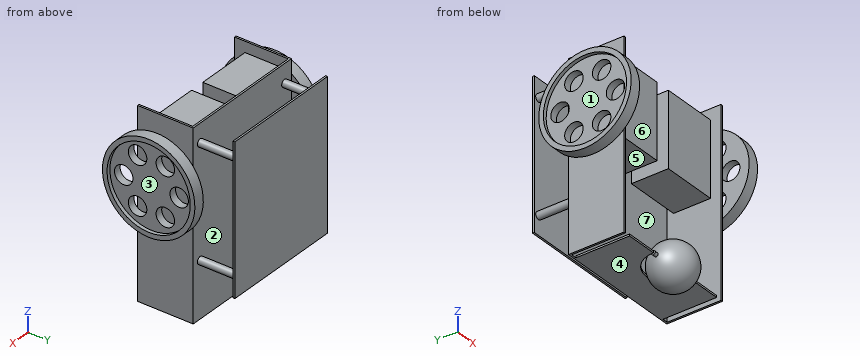
from build123d import *

# Parameters (mm, degrees)
SKETCH_1_W               = 70
SKETCH_1_H               = 100
EXTRUDE_1_DEPTH          = 30
SHELL_1_T                = -1
SKETCH_2_W               = 40
SKETCH_2_H               = 20
EXTRUDE_2_DEPTH          = 30
SKETCH_3_R               = 1.5
EXTRUDE_3_DEPTH          = 10
SKETCH_4_R               = 25
EXTRUDE_4_DEPTH          = 6
SKETCH_5_R               = 22.5
CUT_EXTRUDE_1_DEPTH      = 2
SKETCH_6_R               = 5
CUT_EXTRUDE_2_DEPTH      = 8
PATTERN_CIRCULAR_1_COUNT = 6
MIRROR_1_COPY_1_SKETCH_R = 5
MIRROR_1_COPY_1_DEPTH    = 8
MIRROR_1_COPY_2_SKETCH_R = 5
MIRROR_1_COPY_2_DEPTH    = 8
MIRROR_1_COPY_3_SKETCH_R = 5
MIRROR_1_COPY_3_DEPTH    = 8
MIRROR_1_COPY_4_SKETCH_R = 5
MIRROR_1_COPY_4_DEPTH    = 8
MIRROR_1_COPY_5_SKETCH_R = 5
MIRROR_1_COPY_5_DEPTH    = 8
SKETCH_9_R               = 14
CUT_EXTRUDE_4_DEPTH      = 8
SKETCH_8_W               = 3
SKETCH_8_H               = 29
CUT_EXTRUDE_3_DEPTH      = 8
SKETCH_10_R              = 1
EXTRUDE_5_DEPTH          = 14
SKETCH_11_R              = 2
EXTRUDE_6_DEPTH          = 20
SKETCH_12_W              = 66
SKETCH_12_H              = 80
EXTRUDE_7_DEPTH          = 1


with BuildPart() as part:
    # Sketch 1 → Extrude 1 (new body)
    with BuildSketch(Plane(origin=(0, 0, 0), x_dir=(1, 0, 0), z_dir=(0, 1, 0))):
        with Locations((0, 50)):
            Rectangle(SKETCH_1_W, SKETCH_1_H)
    extrude(amount=EXTRUDE_1_DEPTH)

    # Shell 1
    shell_1_openings = [part.faces().sort_by_distance(p)[0] for p in [
        (0, 0, -50),
        (0, 15, 0),
    ]]
    offset(amount=SHELL_1_T, openings=shell_1_openings, kind=Kind.INTERSECTION)

    # Sketch 2 → Extrude 2 (add)
    with BuildSketch(Plane.ZY.offset(-34)):
        with Locations((-25.793166275, 15.578551741)):
            Rectangle(SKETCH_2_W, SKETCH_2_H)
    extrude_2 = extrude(amount=EXTRUDE_2_DEPTH)

    # Sketch 3 → Extrude 3 (add)
    with BuildSketch(Plane(origin=(35, 0, 0), x_dir=(0, 0, -1), z_dir=(1, 0, 0))):
        with Locations((32, 13.5)):
            Circle(SKETCH_3_R)
    extrude_3 = extrude(amount=EXTRUDE_3_DEPTH)

    # Sketch 4 → Extrude 4 (add)
    with BuildSketch(Plane(origin=(45, 0, 0), x_dir=(0, 0, -1), z_dir=(1, 0, 0))):
        with Locations((32, 13.5)):
            Circle(SKETCH_4_R)
    extrude_4 = extrude(amount=-EXTRUDE_4_DEPTH)

    # Sketch 5 → Cut-Extrude 1 (cut)
    with BuildSketch(Plane(origin=(45, 0, 0), x_dir=(0, 0, -1), z_dir=(1, 0, 0))):
        with Locations((32, 13.5)):
            Circle(SKETCH_5_R)
    cut_extrude_1 = extrude(amount=-CUT_EXTRUDE_1_DEPTH, mode=Mode.SUBTRACT)

    # Sketch 6 → Cut-Extrude 2 (cut)
    with BuildSketch(Plane(origin=(43, 0, 0), x_dir=(0, 0, -1), z_dir=(1, 0, 0))):
        with Locations((32, 28.5)):
            Circle(SKETCH_6_R)
    cut_extrude_2 = extrude(amount=-CUT_EXTRUDE_2_DEPTH, mode=Mode.SUBTRACT)

    # Pattern Circular 1: Cut-Extrude 2 ×6 about axis
    pattern_circular_1_axis = Axis((0, 13.5, -32), (1, 0, 0))
    for i in range(1, PATTERN_CIRCULAR_1_COUNT):
        add(cut_extrude_2.rotate(pattern_circular_1_axis, i * 360 / PATTERN_CIRCULAR_1_COUNT), mode=Mode.SUBTRACT)

    # Mirror 1: Extrude 2, Extrude 3, Extrude 4, Cut-Extrude 1, Cut-Extrude 2 across plane
    add(extrude_2.mirror(Plane(origin=(0, 0, 0), x_dir=(0, 0, 1), z_dir=(1, 0, 0))))
    add(extrude_3.mirror(Plane(origin=(0, 0, 0), x_dir=(0, 0, 1), z_dir=(1, 0, 0))))
    add(extrude_4.mirror(Plane(origin=(0, 0, 0), x_dir=(0, 0, 1), z_dir=(1, 0, 0))))
    add(cut_extrude_1.mirror(Plane(origin=(0, 0, 0), x_dir=(0, 0, 1), z_dir=(1, 0, 0))), mode=Mode.SUBTRACT)
    add(cut_extrude_2.mirror(Plane(origin=(0, 0, 0), x_dir=(0, 0, 1), z_dir=(1, 0, 0))), mode=Mode.SUBTRACT)

    # Mirror 1 copy 1 sketch → Mirror 1 copy 1 (cut)
    with BuildSketch(Plane(origin=(-43, -20.962812921, -27.691342951), x_dir=(0, 0.866025404, -0.5), z_dir=(-1, 0, 0))):
        with Locations((32, -28.5)):
            Circle(MIRROR_1_COPY_1_SKETCH_R)
    extrude(amount=-MIRROR_1_COPY_1_DEPTH, mode=Mode.SUBTRACT)

    # Mirror 1 copy 2 sketch → Mirror 1 copy 2 (cut)
    with BuildSketch(Plane(origin=(-43, -7.462812921, -59.691342951), x_dir=(0, 0.866025404, 0.5), z_dir=(-1, 0, 0))):
        with Locations((32, -28.5)):
            Circle(MIRROR_1_COPY_2_SKETCH_R)
    extrude(amount=-MIRROR_1_COPY_2_DEPTH, mode=Mode.SUBTRACT)

    # Mirror 1 copy 3 sketch → Mirror 1 copy 3 (cut)
    with BuildSketch(Plane(origin=(-43, 27, -64), x_dir=(0, 0, 1), z_dir=(-1, 0, 0))):
        with Locations((32, -28.5)):
            Circle(MIRROR_1_COPY_3_SKETCH_R)
    extrude(amount=-MIRROR_1_COPY_3_DEPTH, mode=Mode.SUBTRACT)

    # Mirror 1 copy 4 sketch → Mirror 1 copy 4 (cut)
    with BuildSketch(Plane(origin=(-43, 47.962812921, -36.308657049), x_dir=(0, -0.866025404, 0.5), z_dir=(-1, 0, 0))):
        with Locations((32, -28.5)):
            Circle(MIRROR_1_COPY_4_SKETCH_R)
    extrude(amount=-MIRROR_1_COPY_4_DEPTH, mode=Mode.SUBTRACT)

    # Mirror 1 copy 5 sketch → Mirror 1 copy 5 (cut)
    with BuildSketch(Plane(origin=(-43, 34.462812921, -4.308657049), x_dir=(0, -0.866025404, -0.5), z_dir=(-1, 0, 0))):
        with Locations((32, -28.5)):
            Circle(MIRROR_1_COPY_5_SKETCH_R)
    extrude(amount=-MIRROR_1_COPY_5_DEPTH, mode=Mode.SUBTRACT)

    # Sketch 9 → Cut-Extrude 4 (cut)
    with BuildSketch(Plane(origin=(0, 0, -100), x_dir=(-1, 0, 0), z_dir=(0, 0, -1))):
        Circle(SKETCH_9_R)
    extrude(amount=-CUT_EXTRUDE_4_DEPTH, mode=Mode.SUBTRACT)

    # Sketch 8 → Cut-Extrude 3 (cut)
    with BuildSketch(Plane(origin=(0, 0, -100), x_dir=(-1, 0, 0), z_dir=(0, 0, -1))):
        with Locations((32.5, 14.5)):
            Rectangle(SKETCH_8_W, SKETCH_8_H)
        with Locations((-32.5, 14.5)):
            Rectangle(SKETCH_8_W, SKETCH_8_H)
    extrude(amount=-CUT_EXTRUDE_3_DEPTH, mode=Mode.SUBTRACT)



with BuildPart() as body_2:
    # Sketch 7 → Revolve 1 (revolve)
    with BuildSketch(Plane(origin=(0, 0, -100), x_dir=(-1, 0, 0), z_dir=(0, 0, -1))):
        with BuildLine():
            Line((-12, 0), (12, 0))
            ThreePointArc((12, 0), (0, 12), (-12, 0))
        make_face()
    revolve(axis=Axis((12, 0, -100), (-1, 0, 0)))


with BuildPart() as part_1:
    add(part.part)

    add(body_2.part)  # Extrude 5 merges body 2
    # Sketch 10 → Extrude 5 (add, symmetric)
    with BuildSketch(Plane(origin=(0, 0, 0), x_dir=(0, 0, -1), z_dir=(1, 0, 0))):
        with Locations((100, 0)):
            Circle(SKETCH_10_R)
    extrude(amount=EXTRUDE_5_DEPTH, both=True)

    # Sketch 11 → Extrude 6 (add)
    with BuildSketch(Plane(origin=(0, 30, 0), x_dir=(1, 0, 0), z_dir=(0, 1, 0))):
        with Locations((30, 70)):
            Circle(SKETCH_11_R)
        with Locations((-30, 70)):
            Circle(SKETCH_11_R)
        with Locations((-30, 10)):
            Circle(SKETCH_11_R)
        with Locations((30, 10)):
            Circle(SKETCH_11_R)
    extrude(amount=EXTRUDE_6_DEPTH)

    # Sketch 12 → Extrude 7 (add)
    with BuildSketch(Plane(origin=(0, 50, 0), x_dir=(1, 0, 0), z_dir=(0, 1, 0))):
        with Locations((0, 40)):
            Rectangle(SKETCH_12_W, SKETCH_12_H)
    extrude(amount=EXTRUDE_7_DEPTH)


solid = part_1.part
Source: CAD feature listing. Evaluate the final solid. Frame: model axes, mm. Face numbers are marked on the shaded views. A direction names the side the tool comes from. Round coordinates to 2 decimals unless told otherwise and drop trailing zeros. Write each loop counter-clockwise with the first axis right and the second up, starting at its lowest first coordinate (ties: lowest second). Pieces come first, ordered by that corner, then holes. Notation, with made-up numbers: (56.25, 80) - (61.25, 80) arc R19 ccw to (61.25, 108) - close; hole circle Ø11 at (-14.5, 42). An arc over 180 degrees is marked (long way). Use CSV: the item, a comma, the result in double quotes. Start each with the question number.
(1) Cut plane A-A, the plane x = -20.5. Return loops of the section in (y, z), and give its area (3 significant figures).
(2) Cut plane B-B, the plane z = -93. Return loops of the section in (x, y).
(3) Material intervals for probe 1 along X at (y, z) = (24, -13); probe 2 along Y at (x, z) = (-16, -20); probe 3 along Y at (x, z) = (-22, -63.5), sorted ascending. Write a range as [from, to].
(4) Set-up query: the marked faces 4, 5, 6 and 7. Return all of +Z, -Z, +X, -X, +Y, -Y with unobstructed straight access to the full face (end or side cutting, diameter ignored); none if empty.
(5) Mould query, pull axis X, two halves, no side actions, for the marked faces 1, 2 and 3. Classes: pulls with the +X half, pulls with the -X half, needs draft (parallel to the pull), parting line crosses it, or undercut.
(6) Cut plane C-C, the plane z = -52. Return loops of the section in (x, y).
(7) Cut plane D-D, the plane y = 40.5. Return loops of the section in (x, z).
(8) First-contact query: pin 1 Ø1 at (x, y) = (0.5, 1) entering from -Z; pin 2 Ø5 at (x, z) = (21, -81.5) entering from +Y; pin 3 Ø14.5 at (y, z) = (21, -68.5) entering from -X; pin 4 Ø1.6 at (y, z) = (0, -100) entering from +X. Flat tips, straight axial feed; report the tip coordinate or a pass-through.
Geometry says:
1,outline,"(0, -100) - (30, -100) - (30, 0) - (29, 0) - (29, -99) - (0, -99) - close; (5.58, -45.79) - (25.58, -45.79) - (25.58, -5.79) - (5.58, -5.79) - close; (50, -80) - (51, -80) - (51, 0) - (50, 0) - close"
1,area,"1,010 mm²"
2,outline,"(-35, 0) - (-34, 0) - (-34, 29) - (34, 29) - (34, 0) - (35, 0) - (35, 30) - (-35, 30) - close; circle Ø19.49 at (0, 0)"
3,probe 1,"[-43, -39], [-35, -4], [4, 35], [39, 43]"
3,probe 2,"[5.58, 25.58], [29, 30], [50, 51]"
3,probe 3,"[29, 30], [50, 51]"
4,face 4,"-Z, +Y"
4,face 5,"-Y"
4,face 6,"+Z, -Y"
4,face 7,"+Z"
5,face 1,"pulls with the -X half"
5,face 2,"undercut"
5,face 3,"pulls with the +X half"
6,outline,"(-45, -1.5) - (-39, -1.5) - (-39, 28.5) - (-45, 28.5) - (-45, 23.81) - (-43, 23.81) - (-43, 3.19) - (-45, 3.19) - close; (-35, 0) - (-34, 0) - (-34, 29) - (34, 29) - (34, 0) - (35, 0) - (35, 30) - (-35, 30) - close; (-33, 50) - (33, 50) - (33, 51) - (-33, 51) - close; (39, -1.5) - (45, -1.5) - (45, 3.19) - (43, 3.19) - (43, 23.81) - (45, 23.81) - (45, 28.5) - (39, 28.5) - close"
7,outline,"circle Ø4 at (-30, -70); circle Ø4 at (-30, -10); circle Ø4 at (30, -70); circle Ø4 at (30, -10)"
8,pin 1,"z = -111.98"
8,pin 2,"y = 51"
8,pin 3,"x = -35"
8,pin 4,"x = 35"
